Geometry: see drawing. Coordinates: mm, zero at the bounding-box minimum. Round coordinates to 2 decimals unless told otherwise and drop trailing zeros. Loops run counter-clockwise (first coordinate to the right, second up) from the corner with the lowest first, then second, coordinate; pieces in that order, holes last. Notation, with made-up numbers: (67, -34.5) - (117, -34.5) arc R19 ccw to (117, -26.5) - close; hole circle Ø4 at (63.25, -12). An arc over 180 degrees is marked (long way). Return JSON: item names as keys, results as strings. Group by question number.
1. Section B-B on z = 0.95. Count the separate pieces of the cut face and the enclosed holes in it, and give its area (3 significant figures).
2. Section A-A on x = 25. Return loops of the section in (y, z).
3. Section C-C on y = 10. Return loops of the section in (x, z).
4. First-contact query: pin 1 Ø16 at (x, y) = (42.32, 15) entering from -Z; pin 2 Ø1 at (y, z) = (29, 1.5) entering from -X; pin 3 Ø1 at (y, z) = (13, 2.5) entering from -X; pin 4 Ø1.5 at (y, z) = (10, 1.5) entering from -X. Flat tips, straight axial feed; report the tip coordinate or a pass-through.
5. Draft query along X for the marked faces 1, 2 and 3. Return one class per face: +X half, -X half, draft (parallel to the pull), parting line (faces both ways), or undercut.
6. Material intervals for probe 1 along X at (y, z) = (23, 0.6); probe 2 along Y at (x, z) = (40, 1.3) (1 decimal); probe 3 along Y at (x, z) = (11.5, 1.85), sorted ascending.
7. Section D-D on x = 39.5. Return loops of the section in (y, z) (1 decimal).
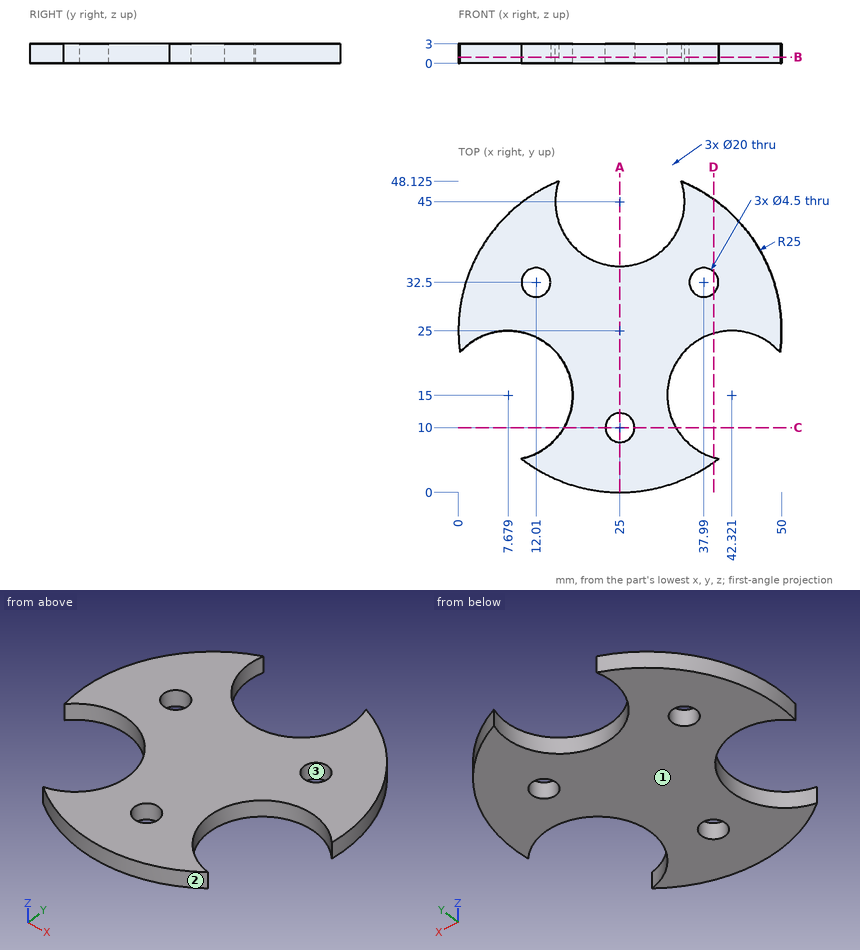
Taken from the geometry:
{
 "1": {"separate pieces": "1", "enclosed holes": "3", "area": "1,190 mm2"},
 "2": {"outline": "(0, 0) - (7.75, 0) - (7.75, 3) - (0, 3) - close; (12.25, 0) - (35, 0) - (35, 3) - (12.25, 3) - close"},
 "3": {"outline": "(16.34, 0) - (22.75, 0) - (22.75, 3) - (16.34, 3) - close; (27.25, 0) - (33.66, 0) - (33.66, 3) - (27.25, 3) - close"},
 "4": {"pin 1": "through", "pin 2": "x = 0.25", "pin 3": "x = 17.36", "pin 4": "x = 15.86"},
 "5": {"face 1": "draft", "face 2": "parting line", "face 3": "undercut"},
 "6": {"probe 1": "0.08 to 1.68, 13.68 to 36.32, 48.32 to 49.92", "probe 2": "5 to 5.3, 24.7 to 31.5, 33.5 to 45", "probe 3": "3.96 to 5.76, 24.24 to 30.31, 34.69 to 46.04"},
 "7": {"outline": "(4.6, 0) - (5.4, 0) - (5.4, 3) - (4.6, 3) - close; (24.6, 0) - (30.8, 0) - (30.8, 3) - (24.6, 3) - close; (34.2, 0) - (45.4, 0) - (45.4, 3) - (34.2, 3) - close"}
}
